Work out the finished part from the listing and answer in its coordinate system (mm). A direction names the side the tool comes from. Coordinates: 2 decimals unless noted, no trailing zeros. Loops run counter-clockwise (first coordinate to the right, second up) from the corner with the lowest first, then second, coordinate; pieces in that order, holes last. Notation, with made-up numbers: (86.25, -2.75) - (112.25, -2.75) arc R13 cw to (112.25, 10.25) - close; hole circle Ø4 at (-8.75, 50.25). An arc over 180 degrees is marked (long way). Write each question's results on one line, items separated by ' | '. Start each with the question number.
1. Determine the mould class of faces 1 (the flat face through (14, 4, 15)), 2 (the cylindrical face through (-23.846, -7.509, 21.888)), 3 (the flat face through (-20, 16, 14)) for opening direction Y: released by +Y, released by -Y, zero draft, split by the parting line, or undercut.
2. Find the intervals of material crossed by line 1 along Z through (x, y) = (22, 0); line 2 along Y through (x, z) = (0, 18.25); line 3 along Z through (x, y) = (-31.5, 36), in increasing order. Write a range as [from, to].
3. Each of these flat-tipped pins is pushed along its axis until it touches: P1, Ø4.5, axis at y = 0, z = 22, coming from the +X side; P2, Ø5, axis at x = -33.5, z = 5, coming from the -Y side; P3, Ø6, axis at y = 8, z = 8, coming from the +X side; P4, Ø1.5, axis at x = -14.5, y = 2.5, coming from the -Z side. Where does it stop, or does it pass through?
4. Which of the six approach directions +Z, -Z, +X, -X, +Y, -Y give full straight-line access (tool end or side, diameter ignored) to faces 4 (the flat face through (15.8, 0, 15)), 5 (the cylindrical face through (20.5, -0.1, 19.5)), 6 (the flat face through (5.9, -11.5, 30))?
5. A cutting plane is placed at A-A on z = 18. Determine the outline of the cut face in (x, y).
from build123d import *

# Parameters (mm, degrees)
EXTRUDE_1_DEPTH     = 14
SKETCH_2_R          = 25
EXTRUDE_2_DEPTH     = 30
SKETCH_3_R          = 12.5
CUT_EXTRUDE_1_DEPTH = 78.64562782
SWEEP_2_PROFILE_R   = 2.5
SKETCH_8_W          = 15.8
SKETCH_8_H          = 8
CUT_EXTRUDE_3_DEPTH = 78.64562782


with BuildPart() as part:
    # 草图1 → 凸台-拉伸1 (new body)
    with BuildSketch(Plane.XY):
        with BuildLine():
            add(Edge.make_bspline(
                [(33, 0), (32.992204895, 0.544666729), (32.976480109, 1.643403319), (32.853064931, 3.301727765), (32.658915426, 4.980879695), (32.388196689, 6.677537715), (32.044944958, 8.388606268), (31.630570565, 10.111165253), (31.147186794, 11.842433965), (30.596568938, 13.57971361), (29.98033344, 15.320337013), (29.299789777, 17.061615147), (28.555887029, 18.800784535), (27.749173646, 20.534967231), (26.879751228, 22.261119957), (25.947286594, 23.976001144), (24.951020471, 25.676125073), (23.889814679, 27.35772059), (22.762223009, 29.016688558), (21.566586312, 30.648565024), (20.301138192, 32.248479161), (18.964127555, 33.81112609), (17.553956129, 35.330754232), (16.069306796, 36.801162963), (14.509273248, 38.215722303), (12.873484417, 39.567416225), (11.162207045, 40.848898292), (9.376441015, 42.052578226), (7.517986505, 43.170717712), (5.589490091, 44.195539218), (3.594469744, 45.119346278), (1.53731504, 45.934646153), (-0.576735961, 46.634276616), (-2.74164203, 47.211518041), (-4.950619716, 47.660204084), (-7.196219851, 47.974828288), (-9.470422571, 48.150607487), (-11.76473259, 48.183580117), (-14.070288761, 48.070629868), (-16.377971366, 47.809547695), (-18.67851562, 47.399040683), (-20.96262116, 46.838742341), (-23.221064088, 46.12921357), (-25.444800735, 45.271912976), (-27.625072088, 44.269170741), (-29.753502784, 43.124146476), (-31.822186889, 41.840759247), (-33.823775568, 40.423630812), (-35.751543622, 38.877994203), (-37.599456194, 37.209613013), (-39.362201277, 35.424668235), (-41.035231852, 33.529668236), (-42.614754199, 31.53132517), (-44.09777446, 29.436479773), (-45.481085646, 27.253115728), (-46.760721786, 24.993714386), (-47.930689696, 22.669528818), (-48.985280232, 20.290366962), (-49.921879744, 17.86233444), (-50.73821056, 15.391267947), (-51.432305812, 12.8831224), (-52.002502766, 10.343940159), (-52.447402955, 7.779839842), (-52.766015438, 5.196990334), (-52.957281079, 2.601648936), (-53.021584789, 0.009188241), (-52.95682309, -2.556762808), (-52.768752296, -5.077096398), (-52.522148692, -6.726622939), (-52.399929, -7.544148)],
                knots=[0, 0, 0, 0, 0.010895628, 0.021979359, 0.033249847, 0.044704843, 0.056341204, 0.068154912, 0.080141086, 0.092294104, 0.104607701, 0.11707519, 0.129689707, 0.14244447, 0.155333078, 0.168349762, 0.181489545, 0.194748369, 0.208123105, 0.221611441, 0.235211792, 0.248923032, 0.26274432, 0.276674885, 0.290713819, 0.304859987, 0.319111923, 0.333467808, 0.347925543, 0.362482829, 0.377137264, 0.391886521, 0.406728484, 0.421661423, 0.436684102, 0.451795886, 0.466996829, 0.482287719, 0.497670025, 0.513145895, 0.528718049, 0.54438967, 0.560164277, 0.576045576, 0.592037302, 0.608143104, 0.624366387, 0.640710242, 0.657177353, 0.673769958, 0.690489849, 0.70733837, 0.724316458, 0.741424727, 0.758663496, 0.776003856, 0.793351474, 0.810699088, 0.828046707, 0.845394323, 0.862741936, 0.880089557, 0.897437174, 0.914784793, 0.932132405, 0.949480024, 0.966642526, 0.983467637, 1, 1, 1, 1], degree=3))
            add(Edge.make_bspline(
                [(-52.399929, -7.544148), (-52.251447511, -8.344449933), (-51.956477891, -9.93430977), (-51.431378847, -11.881327743), (-50.946615492, -13.402352601), (-50.547774852, -14.520833098), (-50.113968755, -15.61972104), (-49.645210909, -16.698158038), (-49.141976069, -17.755310038), (-48.604716766, -18.790320175), (-48.033993716, -19.80233339), (-47.430434687, -20.790495875), (-46.794737646, -21.753963168), (-46.127681435, -22.691905033), (-45.430091118, -23.603527112), (-44.461690461, -24.78142675), (-43.179240858, -26.184980253), (-41.532569131, -27.753864704), (-39.788936475, -29.201085533), (-37.95827815, -30.522875718), (-36.050936512, -31.716585493), (-34.077553488, -32.780697635), (-32.048834528, -33.714886161), (-29.975350706, -34.520036776), (-27.867326416, -35.19822348), (-25.734442747, -35.752653633), (-23.585659114, -36.187574089), (-21.429063355, -36.50814968), (-19.27176002, -36.720310246), (-17.119804246, -36.830595085), (-14.978186003, -36.845970949), (-12.850873113, -36.773654705), (-10.740913687, -36.620937922), (-8.650597875, -36.395022526), (-6.581674525, -36.102863407), (-4.535611161, -35.751026937), (-2.513887786, -35.345556209), (-0.518293788, -34.891856115), (1.448781863, -34.394574738), (3.384105738, -33.857530642), (5.283395004, -33.283637208), (7.141181014, -32.67491492), (8.950717416, -32.03256093), (10.703916152, -31.357116), (12.391331701, -30.648817619), (14.002048983, -29.907900792), (15.525340793, -29.134972637), (16.967203751, -28.319820567), (18.341157037, -27.449470169), (19.665980256, -26.516508819), (20.943385245, -25.51958757), (22.170348028, -24.461209886), (23.343896741, -23.343896621), (24.461208994, -22.170347615), (25.519591016, -20.943387015), (26.516495927, -19.665973587), (27.449518295, -18.341181942), (28.316413718, -16.972205388), (29.115091885, -15.562340777), (29.843629808, -14.114985263), (30.500271052, -12.633625806), (31.083435636, -11.121830348), (31.591710671, -9.583242061), (32.023907296, -8.021566688), (32.37884622, -6.440566847), (32.656192002, -4.844051032), (32.853335771, -3.23586502), (32.977041039, -1.619883695), (32.992347014, -0.539961135), (33, 0)],
                knots=[0, 0, 0, 0, 0.020431005, 0.040587725, 0.050576924, 0.060511834, 0.070396638, 0.08023526, 0.09003139, 0.099788458, 0.109509648, 0.119197921, 0.128855969, 0.138486254, 0.14809097, 0.157672096, 0.176767364, 0.195785952, 0.214735199, 0.233619037, 0.252438345, 0.271191379, 0.289874288, 0.308481685, 0.327007235, 0.345444275, 0.363786425, 0.382028051, 0.400164732, 0.418193505, 0.436112913, 0.453922863, 0.47162413, 0.489217593, 0.50670321, 0.524078705, 0.54133817, 0.558470582, 0.575458641, 0.592277781, 0.60889569, 0.625272245, 0.641359738, 0.657103167, 0.672440382, 0.687301883, 0.701610051, 0.715317718, 0.728874017, 0.74243031, 0.75598661, 0.769542915, 0.783099211, 0.796655507, 0.810211812, 0.823768112, 0.837324405, 0.850880704, 0.86443701, 0.877993308, 0.891549609, 0.905105906, 0.918662207, 0.932218502, 0.945774799, 0.959331099, 0.972887398, 0.986443703, 1, 1, 1, 1], degree=3))
        make_face()
    extrude(amount=EXTRUDE_1_DEPTH)

    # 草图2 → 凸台-拉伸2 (add)
    with BuildSketch(Plane.XY):
        with Locations(Location((0, 0, 0), (0, 0, 180))):
            Circle(SKETCH_2_R)
    extrude(amount=EXTRUDE_2_DEPTH)

    # 草图3 → 切除-拉伸1 (cut, through all)
    with BuildSketch(Plane.XY.offset(30)):
        Circle(SKETCH_3_R)
    extrude(amount=-CUT_EXTRUDE_1_DEPTH, mode=Mode.SUBTRACT)

    # 切除-扫描2: sweep along a curve in space
    with BuildLine() as sweep_2_path:
        Line((0, 0, 22), (27, 0, 22))
    # 切除-扫描2 profile (on start of the path) → 切除-扫描2 (sweep, cut)
    with BuildSketch(Plane(origin=(0, 0, 22), x_dir=(0, 0, 1), z_dir=(1, 0, 0))):
        Circle(SWEEP_2_PROFILE_R)
    sweep(path=sweep_2_path.line, mode=Mode.SUBTRACT)

    # 草图8 → 切除-拉伸3 (cut, through all)
    with BuildSketch(Plane.XY):
        with Locations((7.9, 0)):
            Rectangle(SKETCH_8_W, SKETCH_8_H)
    extrude(amount=CUT_EXTRUDE_3_DEPTH, mode=Mode.SUBTRACT)


solid = part.part
Values:
1) face 1: undercut | face 2: split by the parting line | face 3: zero draft
2) line 1: [0, 19.5], [24.5, 30] | line 2: [-25, -12.5], [12.5, 25] | line 3: [0, 14]
3) P1: x = -12.3 | P2: y = -34.12 | P3: x = 32.64 | P4: z = 0
4) face 4: +Z, -Z | face 5: +X | face 6: +Z, +X, -X, +Y, -Y
5) outline: circle Ø50 at (0, 0); hole (11.84, -4) - (15.8, -4) - (15.8, 4) - (11.84, 4) arc R12.5 ccw (long way) to start
